For this review, take the finished solid that the model builds, in its own axes (mm). Give positions to 0.01 mm unless a question says otherwise; leave off trailing zeros. Loops run counter-clockwise (first coordinate to the right, second up) from the corner with the lowest first, then second, coordinate; pieces in that order, holes last.
```python
from build123d import *

# Parameters (mm, degrees)
SKETCH1_W           = 38.1
SKETCH1_H           = 88.9
BOSS_EXTRUDE1_DEPTH = 2362.2
SKETCH2_R           = 21.43125
CUT_EXTRUDE4_DEPTH  = 2363.925359062
FILLET1_R           = 3.175


with BuildPart() as part:
    # Sketch1 → Boss-Extrude1 (new body)
    with BuildSketch(Plane(origin=(0, 0, 0), x_dir=(1, 0, 0), z_dir=(0, 1, 0))):
        Rectangle(SKETCH1_W, SKETCH1_H)
    extrude(amount=BOSS_EXTRUDE1_DEPTH)

    # Sketch2 → Cut-Extrude4 (cut, through all)
    with BuildSketch(Plane(origin=(-19.05, 0, 0), x_dir=(0, 0, -1), z_dir=(1, 0, 0))):
        with Locations(Location((12.7, 458.7875, 0), (0, 0, 180))):
            Circle(SKETCH2_R)
        with Locations(Location((12.7, 939.8, 0), (0, 0, 180))):
            Circle(SKETCH2_R)
    cut_extrude4 = extrude(amount=CUT_EXTRUDE4_DEPTH, mode=Mode.SUBTRACT)

    # Fillet1
    fillet1_edges = [part.edges().sort_by_distance(p)[0] for p in [
        (19.05, 1181.1, 44.45),
        (-19.05, 1181.1, 44.45),
        (-19.05, 1181.1, -44.45),
        (19.05, 1181.1, -44.45),
    ]]
    fillet(fillet1_edges, radius=FILLET1_R)

    # Mirror1: Cut-Extrude4 across plane
    add(cut_extrude4.mirror(Plane(origin=(0, 1181.1, 0), x_dir=(0, 0, 1), z_dir=(0, -1, 0))), mode=Mode.SUBTRACT)


solid = part.part
```
Q1. For probe 1 along Y at (x, z) = (-13, -15); probe 2 along Y at (x, z) = (-7, -12.7); probe 3 along Z at (x, y) = (3, 939), list the stretches that pass through material, from the lowest coordinate up.
Answers:
probe 1: y = 0 to 437.48, 480.09 to 918.49, 961.11 to 1401.09, 1443.71 to 1882.11, 1924.72 to 2362.2
probe 2: y = 0 to 437.36, 480.22 to 918.37, 961.23 to 1400.97, 1443.83 to 1881.98, 1924.84 to 2362.2
probe 3: z = -44.45 to -34.12, 8.72 to 44.45
Q2. Consider section B-B on y = 939.8. Give the boundary of the cut face in (x, z) (3 decimals), plus the area to 3 significant figures.
Answers:
outline: (-19.05, -41.275) arc R3.175 ccw to (-15.875, -44.45) - (15.875, -44.45) arc R3.175 ccw to (19.05, -41.275) - (19.05, -34.131) - (-19.05, -34.131) - close; (-19.05, 8.731) - (19.05, 8.731) - (19.05, 41.275) arc R3.175 ccw to (15.875, 44.45) - (-15.875, 44.45) arc R3.175 ccw to (-19.05, 41.275) - close
area: 1,750 mm2
Q3. Consider section A-A on z = -12.7. Give the boundary of the cut face in (x, y), plus the area to 3 significant figures.
Answers:
outline: (-19.05, 0) - (19.05, 0) - (19.05, 437.36) - (-19.05, 437.36) - close; (-19.05, 480.22) - (19.05, 480.22) - (19.05, 918.37) - (-19.05, 918.37) - close; (-19.05, 961.23) - (19.05, 961.23) - (19.05, 1400.97) - (-19.05, 1400.97) - close; (-19.05, 1443.83) - (19.05, 1443.83) - (19.05, 1881.98) - (-19.05, 1881.98) - close; (-19.05, 1924.84) - (19.05, 1924.84) - (19.05, 2362.2) - (-19.05, 2362.2) - close
area: 83,500 mm2
Q4. For pin 1 Ø1 at (x, z) = (10, 10.5) entering from -Y, flat-tipped, find the tip position at first contact; note if it passes through.
Answers:
pin 1: stops at y = 0
Q5. Mouldability with a two-part tool opening along Z and no side actions: class faces 1 (the flat face through (0, 2362.2, -1)), 2 (the cylindrical face through (-0.27, 1884.4, -2.81)) as +Z half, -Z half, draft (parallel to the pull), parting line (faces both ways), or undercut.
Answers:
face 1: draft
face 2: undercut
